Check sheet for the modelled part. Datum: model origin and axes. Units: mm. Give positions to 0.01 mm unless a question says otherwise; leave off trailing zeros. Loops run counter-clockwise (first coordinate to the right, second up) from the corner with the lowest first, then second, coordinate; pieces in that order, holes last. Notation, with made-up numbers: M 40,51 L 50,51 A23 ccw 50,72 Z; hole C -39,39.25 d2. An arc over 180 degrees is marked long. Write each question's results on one line, items separated by ' | '. Start each with the question number.
1. Sectioned sample at B-B on z = -44. Record the cut outline in (x, y) (3 decimals).
2. Sectioned sample at D-D on y = 2.05. Give the number of separate pieces and of enclosed holes in the cut face, and give its area (3 significant figures).
3. Material ranges on line 1 along X through (y, z) = (0.65, -13.5) (3 decimals); line 2 along Z through (x, y) = (-8, 0.8); line 3 along X through (y, z) = (2.6, -9.5), recorded low to high.
4. Sectioned sample at A-A on x = -30. Record the cut outline in (y, z) (3 decimals), and give its area (4 significant figures).
5. Go/stop test with flat-tipped pins: pin 1 (1.7 mm diameter, centred on x = -8, z = -51.44, fed in from -Y); pin 2 (1.2 mm diameter, centred on y = 1.5, z = -53, fed in from -X); pin 3 (0.8 mm diameter, centred on y = 1, z = -2, fed in from -X). Record where each tip stops, or that it passes through.
6. Sectioned sample at C-C on x = -61.47. Record the cut outline in (y, z), and give its area (3 significant figures).
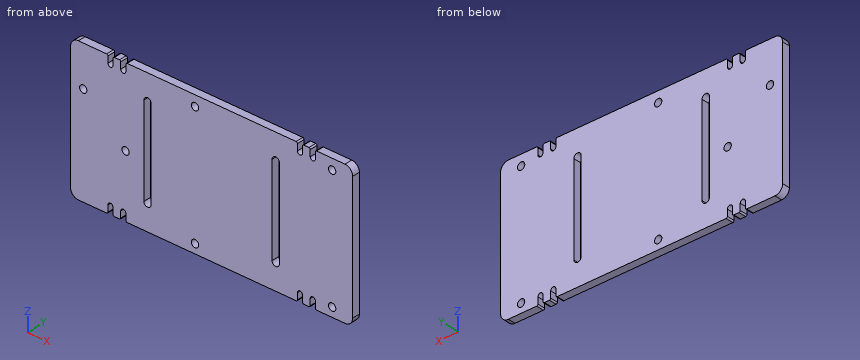
Autodesk Inventor part; units mm, degrees
ref_plane "YZ Plane" through (0, 0, 0) normal (1, 0, 0) x (0, 1, 0)
ref_plane "XZ Plane" through (0, 0, 0) normal (0, 1, 0) x (-1, 0, 0)
ref_plane "XY Plane" through (0, 0, 0) normal (0, 0, 1) x (1, 0, 0)
sketch "Sketch1" plane through (0, 0, 0) normal (0, 1, 0) x (-1, 0, 0)
  line L0 (0, 0) -> (110, 0)
  line L1 (110, 0) -> (110, -55)
  line L2 (110, -55) -> (0, -55)
  line L3 (0, -55) -> (0, 0)
  line L4 (55, 0) -> (55, -55) construction
  circle A0 centre (8, -4.1151) radius 1.425
  circle A1 centre (8, -51.4351) radius 1.425
  circle A2 centre (61.47, -4.1151) radius 1.425
  circle A3 centre (61.47, -51.4351) radius 1.425
  line L5 (8, -4.1151) -> (61.47, -4.1151) construction
  line L6 (61.47, -4.1151) -> (61.47, -51.4351) construction
  line L7 (61.47, -51.4351) -> (8, -51.4351) construction
  line L8 (8, -51.4351) -> (8, -4.1151) construction
  line L9 (80, -10) -> (80, -45) construction
  line L10 (78.575, -10) -> (78.575, -45)
  line L11 (81.425, -45) -> (81.425, -10)
  arc A4 (81.425, -10) -> (78.575, -10) centre (80, -10) ccw
  arc A5 (78.575, -45) -> (81.425, -45) centre (80, -45) ccw
  line L12 (30, -10) -> (30, -45) construction
  line L13 (28.575, -10) -> (28.575, -45)
  line L14 (31.425, -45) -> (31.425, -10)
  arc A6 (31.425, -10) -> (28.575, -10) centre (30, -10) ccw
  arc A7 (28.575, -45) -> (31.425, -45) centre (30, -45) ccw
  circle A8 centre (105.075, -15.8851) radius 1.425
  circle A9 centre (88.565, -30.4901) radius 1.425
  line L15 (108, -12.9601) -> (86.41, -12.9601) construction
  line L16 (86.41, -12.9601) -> (86.41, -43.4401) construction
  line L17 (86.41, -43.4401) -> (108, -43.4401) construction
  line L18 (108, -43.4401) -> (108, -12.9601) construction
  line L19 (105.075, -15.8851) -> (108, -15.8851) construction
  line L20 (105.075, -15.8851) -> (105.075, -12.9601) construction
  point P0 (80, -27.5)
  point P1 (30, -27.5)
  point P2 (55, -27.5)
  dimension "d4" = 53.47
  dimension "d5" = 47.32
  dimension "d12" = 1.425
  dimension "d13" = 50
  dimension "d14" = 2.85
  dimension "d15" = 14.605
  dimension "d16" = 16.51
  dimension "d17" = 21.59
  dimension "d18" = 30.48
  dimension "d19" = 2.925
  dimension "d20" = 8
  dimension "d21" = 2
  dimension "d22" = 55
  dimension "d23" = 110
  dimension "d34" = 35
extrude "Extrusion1" add sketch "Sketch1" along normal blind 3
fillet "Fillet1" radius 3 4 edges at (0, 1.5, -55) (-110, 1.5, -55) (0, 1.5, 0) (-110, 1.5, 0)
sketch "Sketch2" plane through (0, 0, 0) normal (0, -1, 0) x (1, 0, 0)
  arc A0 (-28.575, -10) -> (-31.425, -10) centre (-30, -10) ccw
  line L0 (-28.575, -10) -> (-28.575, -45)
  arc A1 (-31.425, -45) -> (-28.575, -45) centre (-30, -45) ccw
  line L1 (-31.425, -45) -> (-31.425, -10)
  arc A2 (-78.575, -10) -> (-81.425, -10) centre (-80, -10) ccw
  line L2 (-78.575, -10) -> (-78.575, -45)
  arc A3 (-81.425, -45) -> (-78.575, -45) centre (-80, -45) ccw
  line L3 (-81.425, -45) -> (-81.425, -10)
  circle A4 centre (-88.565, -30.4901) radius 1.425
  circle A5 centre (-105.075, -15.8851) radius 1.425
  circle A6 centre (-61.47, -51.4351) radius 1.425
  circle A7 centre (-61.47, -4.1151) radius 1.425
  circle A8 centre (-8, -51.4351) radius 1.425
  circle A9 centre (-8, -4.1151) radius 1.425
  arc A10 (-107, 0) -> (-110, -3) centre (-107, -3) ccw
  line L4 (-110, -3) -> (-110, -52)
  arc A11 (-110, -52) -> (-107, -55) centre (-107, -52) ccw
  line L5 (-107, -55) -> (-3, -55)
  arc A12 (-3, -55) -> (0, -52) centre (-3, -52) ccw
  line L6 (0, -52) -> (0, -3)
  arc A13 (0, -3) -> (-3, 0) centre (-3, -3) ccw
  line L7 (-3, 0) -> (-107, 0)
  line L8 (-107, 0) -> (-3, 0)
  circle A14 centre (-20.937, 0) radius 1.5
  line L9 (-3, -55) -> (-107, -55)
  line L10 (-55, -55) -> (-55, 0) construction
  line L11 (-110, -52) -> (-110, -3)
  line L12 (-110, -27.5) -> (0, -27.5) construction
  circle A15 centre (-15.937, 0) radius 1.5
  circle A16 centre (-89.063, 0) radius 1.5
  circle A17 centre (-94.063, 0) radius 1.5
  circle A18 centre (-20.937, -55) radius 1.5
  circle A19 centre (-15.937, -55) radius 1.5
  circle A20 centre (-89.063, -55) radius 1.5
  circle A21 centre (-94.063, -55) radius 1.5
  point P0 (0, 0)
  dimension "d24" = 3
  dimension "d27" = 5
extrude "Extrusion2" [suppressed]
sketch "Sketch3" plane through (0, 0, 0) normal (0, -1, 0) x (1, 0, 0)
  line L0 (-3, 0) -> (-107, 0)
  line L1 (0, -52) -> (0, -3)
  line L2 (-107, -55) -> (-3, -55)
  line L3 (-110, -3) -> (-110, -52)
  circle A0 centre (-20.551, -3) radius 1
  circle A1 centre (-15.551, -3) radius 1
  line L4 (-21.551, -3) -> (-21.551, 0)
  line L5 (-19.551, -3) -> (-19.551, 0)
  line L6 (-16.551, -3) -> (-16.551, 0)
  line L7 (-14.551, -3) -> (-14.551, 0)
  point P0 (0, 0)
  dimension "d28" = 2
  dimension "d29" = 5
  dimension "d30" = 3
extrude "Extrusion3" cut sketch "Sketch3" against normal through all
ref_plane "Work Plane1" through (-107, 0, -27.5) normal (0, 0, 1) x (1, 0, 0)
ref_plane "Work Plane2" through (-55, 0, -3) normal (1, 0, 0) x (0, 0, -1)
mirror "Mirror1" about plane through (-107, 0, -27.5) normal (0, 0, 1) of "Extrusion3"
mirror "Mirror2" about plane through (-55, 0, -3) normal (1, 0, 0) of "Extrusion3", "Mirror1"
fillet "Fillet2" radius 0.5 16 edges at (-21.551, 1.5, 0) (-19.551, 1.5, 0) (-16.551, 1.5, 0) (-14.551, 1.5, 0) (-14.551, 1.5, -55) (-16.551, 1.5, -55) (-19.551, 1.5, -55) (-21.551, 1.5, -55) (-88.449, 1.5, -55) (-90.449, 1.5, -55) (-93.449, 1.5, -55) (-95.449, 1.5, -55) (-95.449, 1.5, 0) (-93.449, 1.5, 0) (-90.449, 1.5, 0) (-88.449, 1.5, 0)
properties part number "electronics_pouch" material "Wood (Birch)"
Output values:
1) outline: M -110,0 L -81.425,0 L -81.425,3 L -110,3 Z; M -78.575,0 L -31.425,0 L -31.425,3 L -78.575,3 Z; M -28.575,0 L 0,0 L 0,3 L -28.575,3 Z
2) separate pieces: 1 | enclosed holes: 8 | area: 5,730 mm2
3) line 1: -110 to -81.425, -78.575 to -31.425, -28.575 to 0 | line 2: -55 to -52.86, -50.01 to -5.54, -2.69 to 0 | line 3: -110 to -81.33, -78.67 to -31.33, -28.67 to 0
4) outline: M 0,-55 L 3,-55 L 3,-46.425 L 0,-46.425 Z; M 0,-8.575 L 3,-8.575 L 3,0 L 0,0 Z | area: 51.45 mm2
5) pin 1: through | pin 2: x = -109.97 | pin 3: x = -109.94
6) outline: M 0,-55 L 3,-55 L 3,-52.86 L 0,-52.86 Z; M 0,-50.01 L 3,-50.01 L 3,-5.54 L 0,-5.54 Z; M 0,-2.69 L 3,-2.69 L 3,0 L 0,0 Z | area: 148 mm2
